from build123d import *

# Parameters (mm, degrees)
SKETCH1_W           = 60
SKETCH1_H           = 60
BOSS_EXTRUDE1_DEPTH = 5
SKETCH2_W           = 30
SKETCH2_H           = 14.2
SKETCH2_W_2         = 20.2
SKETCH2_H_2         = 8.2
BOSS_EXTRUDE2_DEPTH = 3
SKETCH3_W           = 20.2
SKETCH3_H           = 8.2
CUT_EXTRUDE1_DEPTH  = 15
SKETCH5_R           = 1
CUT_EXTRUDE2_DEPTH  = 15
FILLET1_R           = 2
SKETCH6_W           = 120.017280655
SKETCH6_H           = 101.423054075
CUT_EXTRUDE3_DEPTH  = 15
BOSS_EXTRUDE3_DEPTH = 5
CUT_EXTRUDE4_DEPTH  = 15
FILLET3_R           = 5
SKETCH9_R           = 1
CUT_EXTRUDE5_DEPTH  = 15
SKETCH10_R          = 1
CUT_EXTRUDE6_DEPTH  = 10
FILLET4_R           = 1


with BuildPart() as part:
    # Sketch1 → Boss-Extrude1 (new body)
    with BuildSketch(Plane.XY):
        with Locations((30, 30)):
            Rectangle(SKETCH1_W, SKETCH1_H)
    extrude(amount=BOSS_EXTRUDE1_DEPTH)

    # Sketch2 → Boss-Extrude2 (add)
    with BuildSketch(Plane.XY.offset(5)):
        with Locations((24, 30)):
            Rectangle(SKETCH2_W, SKETCH2_H)
        with Locations((24, 30)):
            Rectangle(SKETCH2_W_2, SKETCH2_H_2, mode=Mode.SUBTRACT)
    extrude(amount=BOSS_EXTRUDE2_DEPTH)

    # Sketch3 → Cut-Extrude1 (cut)
    with BuildSketch(Plane.XY.offset(5)):
        with Locations((24, 30)):
            Rectangle(SKETCH3_W, SKETCH3_H)
    extrude(amount=-CUT_EXTRUDE1_DEPTH, mode=Mode.SUBTRACT)

    # Sketch5 → Cut-Extrude2 (cut)
    with BuildSketch(Plane.XY.offset(8)):
        with Locations((12, 30)):
            Circle(SKETCH5_R)
        with Locations((36, 30)):
            Circle(SKETCH5_R)
    extrude(amount=-CUT_EXTRUDE2_DEPTH, mode=Mode.SUBTRACT)

    # Fillet1
    fillet1_edges = [part.edges().sort_by_distance(p)[0] for p in [
        (39, 22.9, 6.5),
        (39, 37.1, 6.5),
        (9, 37.1, 6.5),
        (9, 22.9, 6.5),
        (0, 0, 2.5),
        (0, 60, 2.5),
        (60, 60, 2.5),
        (60, 0, 2.5),
    ]]
    fillet(fillet1_edges, radius=FILLET1_R)

    # Sketch6 → Cut-Extrude3 (cut)
    with BuildSketch(Plane(origin=(0, 0, 0), x_dir=(-1, 0, 0), z_dir=(0, 0, -1))):
        with Locations((-31.690384235, 31.655167897)):
            Rectangle(SKETCH6_W, SKETCH6_H)
        Polygon((-8.786796564, 51.213203436), (12.426406871, 30), (-30, -12.426406871), (-72.426406871, 30), (-30, 72.426406871), align=None, mode=Mode.SUBTRACT)
    extrude(amount=-CUT_EXTRUDE3_DEPTH, mode=Mode.SUBTRACT)

    # Sketch7 → Boss-Extrude3 (add)
    with BuildSketch(Plane(origin=(0, 0, 0), x_dir=(-1, 0, 0), z_dir=(0, 0, -1))):
        Polygon((-8.786796564, 51.213203436), (12.426406871, 30), (-30, -12.426406871), (-72.426406871, 30), (-30, 72.426406871), align=None)
        Polygon((-19.393398282, 40.606601718), (-8.786796564, 30), (-30, 8.786796564), (-51.213203436, 30), (-30, 51.213203436), align=None, mode=Mode.SUBTRACT)
    extrude(amount=-BOSS_EXTRUDE3_DEPTH)

    # Sketch8 → Cut-Extrude4 (cut)
    with BuildSketch(Plane(origin=(0, 0, 0), x_dir=(-1, 0, 0), z_dir=(0, 0, -1))):
        Polygon((-30, -12.426406871), (12.426406871, 30), (-30, 72.426406871), (-72.426406871, 30), align=None)
        Polygon((-30, -5.355339059), (5.355339059, 30), (-30, 65.355339059), (-65.355339059, 30), align=None, mode=Mode.SUBTRACT)
    extrude(amount=-CUT_EXTRUDE4_DEPTH, mode=Mode.SUBTRACT)

    # Fillet3
    fillet3_edges = [part.edges().sort_by_distance(p)[0] for p in [
        (65.355339059, 30, 2.5),
        (30, 65.355339059, 2.5),
        (-5.355339059, 30, 2.5),
        (30, -5.355339059, 2.5),
    ]]
    fillet(fillet3_edges, radius=FILLET3_R)

    # Sketch9 → Cut-Extrude5 (cut)
    with BuildSketch(Plane(origin=(0, 0, 0), x_dir=(-1, 0, 0), z_dir=(0, 0, -1))):
        with Locations((-30, 58.284271247)):
            Circle(SKETCH9_R)
        with Locations((-30, 1.715728753)):
            Circle(SKETCH9_R)
        with Locations((-1.715728753, 30)):
            Circle(SKETCH9_R)
        with Locations((-58.284271247, 30)):
            Circle(SKETCH9_R)
    extrude(amount=-CUT_EXTRUDE5_DEPTH, mode=Mode.SUBTRACT)

    # Sketch10 → Cut-Extrude6 (cut)
    with BuildSketch(Plane(origin=(0, 0, 0), x_dir=(-1, 0, 0), z_dir=(0, 0, -1))):
        with Locations((-45.556349186, 45.556349186)):
            Circle(SKETCH10_R)
        with Locations((-45.556349186, 14.443650814)):
            Circle(SKETCH10_R)
        with Locations((-14.443650814, 14.443650814)):
            Circle(SKETCH10_R)
        with Locations((-14.443650814, 45.556349186)):
            Circle(SKETCH10_R)
    extrude(amount=-CUT_EXTRUDE6_DEPTH, mode=Mode.SUBTRACT)

    # Fillet4
    # the kernel refuses this fillet: 1 mm, written as the material it adds along each edge
    with BuildSketch(Plane(origin=(37, 35.1, 5), x_dir=(0, 1, 0), z_dir=(-1, 0, 0))) as fillet4_piece_1:
        with BuildLine():
            CenterArc((2 + FILLET4_R, -FILLET4_R), FILLET4_R, 90, 90)
            Line((2, -FILLET4_R), (2, 0))
            Line((2, 0), (2 + FILLET4_R, 0))
        make_face()
    revolve(axis=Axis((37, 35.1, 5), (0, 0, -1)), revolution_arc=90)
    with BuildSketch(Plane(origin=(37, 22.9, 5), x_dir=(0, -1, 0), z_dir=(-1, 0, 0)), Plane(origin=(11, 37.1, 5), x_dir=(0, 1, 0), z_dir=(1, 0, 0))) as fillet4_piece_2:
        with BuildLine():
            CenterArc((FILLET4_R, FILLET4_R), FILLET4_R, 180, 90)
            Line((0, FILLET4_R), (0, 0))
            Line((0, 0), (FILLET4_R, 0))
        make_face()
    extrude(amount=26)
    with BuildSketch(Plane(origin=(9, 24.9, 5), x_dir=(-1, 0, 0), z_dir=(0, 1, 0)), Plane(origin=(39, 35.1, 5), x_dir=(1, 0, 0), z_dir=(0, -1, 0))) as fillet4_piece_3:
        with BuildLine():
            CenterArc((FILLET4_R, FILLET4_R), FILLET4_R, 180, 90)
            Line((0, FILLET4_R), (0, 0))
            Line((0, 0), (FILLET4_R, 0))
        make_face()
    extrude(amount=10.2)
    with BuildSketch(Plane(origin=(11, 24.9, 5), x_dir=(0, -1, 0), z_dir=(1, 0, 0))) as fillet4_piece_4:
        with BuildLine():
            CenterArc((2 + FILLET4_R, -FILLET4_R), FILLET4_R, 90, 90)
            Line((2, -FILLET4_R), (2, 0))
            Line((2, 0), (2 + FILLET4_R, 0))
        make_face()
    revolve(axis=Axis((11, 24.9, 5), (0, 0, -1)), revolution_arc=90)
    with BuildSketch(Plane(origin=(11, 35.1, 5), x_dir=(0, 1, 0), z_dir=(1, 0, 0))) as fillet4_piece_5:
        with BuildLine():
            CenterArc((2 + FILLET4_R, FILLET4_R), FILLET4_R, 180, 90)
            Line((2, FILLET4_R), (2, 0))
            Line((2, 0), (2 + FILLET4_R, 0))
        make_face()
    revolve(axis=Axis((11, 35.1, 5), (0, 0, 1)), revolution_arc=90)
    with BuildSketch(Plane(origin=(37, 24.9, 5), x_dir=(1, 0, 0), z_dir=(0, 1, 0))) as fillet4_piece_6:
        with BuildLine():
            CenterArc((2 + FILLET4_R, -FILLET4_R), FILLET4_R, 90, 90)
            Line((2, -FILLET4_R), (2, 0))
            Line((2, 0), (2 + FILLET4_R, 0))
        make_face()
    revolve(axis=Axis((37, 24.9, 5), (0, 0, -1)), revolution_arc=90)
    # the kernel refuses this fillet: 1 mm, written as the material it takes off along each edge
    with BuildSketch(Plane(origin=(34.1, 25.9, 8), x_dir=(0, 0, -1), z_dir=(0, 1, 0)), Plane(origin=(13.9, 34.1, 8), x_dir=(0, 0, -1), z_dir=(0, -1, 0))) as fillet4_2_piece_1:
        with BuildLine():
            CenterArc((FILLET4_R, -FILLET4_R), FILLET4_R, 90, 90)
            Line((0, -FILLET4_R), (0, 0))
            Line((0, 0), (FILLET4_R, 0))
        make_face()
    extrude(amount=8.2, mode=Mode.SUBTRACT)
    with BuildSketch(Plane(origin=(34.1, 34.1, 8), x_dir=(0, 0, -1), z_dir=(-1, 0, 0)), Plane(origin=(13.9, 25.9, 8), x_dir=(0, 0, -1), z_dir=(1, 0, 0))) as fillet4_2_piece_2:
        with BuildLine():
            CenterArc((FILLET4_R, -FILLET4_R), FILLET4_R, 90, 90)
            Line((0, -FILLET4_R), (0, 0))
            Line((0, 0), (FILLET4_R, 0))
        make_face()
    extrude(amount=20.2, mode=Mode.SUBTRACT)
    with BuildSketch(Plane(origin=(13.9, 25.9, 8), x_dir=(0, 0, -1), z_dir=(1, 0, 0))) as fillet4_2_piece_3a_section:
        with BuildLine():
            CenterArc((FILLET4_R, -FILLET4_R), FILLET4_R, 90, 90)
            Line((0, -FILLET4_R), (0, 0))
            Line((0, 0), (FILLET4_R, 0))
        make_face()
    fillet4_2_piece_3a = extrude(amount=22.7, mode=Mode.PRIVATE)
    fillet4_2_piece_3a = split(fillet4_2_piece_3a, bisect_by=Plane(origin=(34.1, 25.673604886, 7.773604886), z_dir=(1, 0, 0)), keep=Keep.TOP, mode=Mode.PRIVATE)
    with BuildSketch(Plane(origin=(34.1, 23.4, 8), x_dir=(0, 0, -1), z_dir=(0, 1, 0))) as fillet4_2_piece_3b_section:
        with BuildLine():
            CenterArc((FILLET4_R, -FILLET4_R), FILLET4_R, 90, 90)
            Line((0, -FILLET4_R), (0, 0))
            Line((0, 0), (FILLET4_R, 0))
        make_face()
    fillet4_2_piece_3b = extrude(amount=10.7, mode=Mode.PRIVATE)
    fillet4_2_piece_3b = split(fillet4_2_piece_3b, bisect_by=Plane(origin=(34.326395114, 25.9, 7.773604886), z_dir=(0, -1, 0)), keep=Keep.TOP, mode=Mode.PRIVATE)
    fillet4_2_piece_3 = fillet4_2_piece_3a & fillet4_2_piece_3b
    add(fillet4_2_piece_3, mode=Mode.SUBTRACT)
    with BuildSketch(Plane(origin=(34.1, 25.9, 8), x_dir=(0, 0, -1), z_dir=(0, 1, 0))) as fillet4_2_piece_4a_section:
        with BuildLine():
            CenterArc((FILLET4_R, -FILLET4_R), FILLET4_R, 90, 90)
            Line((0, -FILLET4_R), (0, 0))
            Line((0, 0), (FILLET4_R, 0))
        make_face()
    fillet4_2_piece_4a = extrude(amount=10.7, mode=Mode.PRIVATE)
    fillet4_2_piece_4a = split(fillet4_2_piece_4a, bisect_by=Plane(origin=(34.326395114, 34.1, 7.773604886), z_dir=(0, 1, 0)), keep=Keep.TOP, mode=Mode.PRIVATE)
    with BuildSketch(Plane(origin=(36.6, 34.1, 8), x_dir=(0, 0, -1), z_dir=(-1, 0, 0))) as fillet4_2_piece_4b_section:
        with BuildLine():
            CenterArc((FILLET4_R, -FILLET4_R), FILLET4_R, 90, 90)
            Line((0, -FILLET4_R), (0, 0))
            Line((0, 0), (FILLET4_R, 0))
        make_face()
    fillet4_2_piece_4b = extrude(amount=22.7, mode=Mode.PRIVATE)
    fillet4_2_piece_4b = split(fillet4_2_piece_4b, bisect_by=Plane(origin=(34.1, 34.326395114, 7.773604886), z_dir=(1, 0, 0)), keep=Keep.TOP, mode=Mode.PRIVATE)
    fillet4_2_piece_4 = fillet4_2_piece_4a & fillet4_2_piece_4b
    add(fillet4_2_piece_4, mode=Mode.SUBTRACT)
    with BuildSketch(Plane(origin=(13.9, 36.6, 8), x_dir=(0, 0, -1), z_dir=(0, -1, 0))) as fillet4_2_piece_5a_section:
        with BuildLine():
            CenterArc((FILLET4_R, -FILLET4_R), FILLET4_R, 90, 90)
            Line((0, -FILLET4_R), (0, 0))
            Line((0, 0), (FILLET4_R, 0))
        make_face()
    fillet4_2_piece_5a = extrude(amount=10.7, mode=Mode.PRIVATE)
    fillet4_2_piece_5a = split(fillet4_2_piece_5a, bisect_by=Plane(origin=(13.673604886, 34.1, 7.773604886), z_dir=(0, 1, 0)), keep=Keep.TOP, mode=Mode.PRIVATE)
    with BuildSketch(Plane(origin=(34.1, 34.1, 8), x_dir=(0, 0, -1), z_dir=(-1, 0, 0))) as fillet4_2_piece_5b_section:
        with BuildLine():
            CenterArc((FILLET4_R, -FILLET4_R), FILLET4_R, 90, 90)
            Line((0, -FILLET4_R), (0, 0))
            Line((0, 0), (FILLET4_R, 0))
        make_face()
    fillet4_2_piece_5b = extrude(amount=22.7, mode=Mode.PRIVATE)
    fillet4_2_piece_5b = split(fillet4_2_piece_5b, bisect_by=Plane(origin=(13.9, 34.326395114, 7.773604886), z_dir=(-1, 0, 0)), keep=Keep.TOP, mode=Mode.PRIVATE)
    fillet4_2_piece_5 = fillet4_2_piece_5a & fillet4_2_piece_5b
    add(fillet4_2_piece_5, mode=Mode.SUBTRACT)
    with BuildSketch(Plane(origin=(11.4, 25.9, 8), x_dir=(0, 0, -1), z_dir=(1, 0, 0))) as fillet4_2_piece_6a_section:
        with BuildLine():
            CenterArc((FILLET4_R, -FILLET4_R), FILLET4_R, 90, 90)
            Line((0, -FILLET4_R), (0, 0))
            Line((0, 0), (FILLET4_R, 0))
        make_face()
    fillet4_2_piece_6a = extrude(amount=22.7, mode=Mode.PRIVATE)
    fillet4_2_piece_6a = split(fillet4_2_piece_6a, bisect_by=Plane(origin=(13.9, 25.673604886, 7.773604886), z_dir=(-1, 0, 0)), keep=Keep.TOP, mode=Mode.PRIVATE)
    with BuildSketch(Plane(origin=(13.9, 34.1, 8), x_dir=(0, 0, -1), z_dir=(0, -1, 0))) as fillet4_2_piece_6b_section:
        with BuildLine():
            CenterArc((FILLET4_R, -FILLET4_R), FILLET4_R, 90, 90)
            Line((0, -FILLET4_R), (0, 0))
            Line((0, 0), (FILLET4_R, 0))
        make_face()
    fillet4_2_piece_6b = extrude(amount=10.7, mode=Mode.PRIVATE)
    fillet4_2_piece_6b = split(fillet4_2_piece_6b, bisect_by=Plane(origin=(13.673604886, 25.9, 7.773604886), z_dir=(0, -1, 0)), keep=Keep.TOP, mode=Mode.PRIVATE)
    fillet4_2_piece_6 = fillet4_2_piece_6a & fillet4_2_piece_6b
    add(fillet4_2_piece_6, mode=Mode.SUBTRACT)


solid = part.part
Input: part model. Units: mm. Frame: model coordinates. A direction names the side the tool comes from. Coordinates: 2 decimals unless noted, no trailing zeros. Loops run counter-clockwise (first coordinate to the right, second up) from the corner with the lowest first, then second, coordinate; pieces in that order, holes last.
(1) Section D-D on y = 12. Return the cut outline in (x, z), then the cut area to 3 significant figures.
(2) Set-up query: faces 5 (the face through (24, 22.9, 7)), 6 (the face through (9.6, 36.53, 7.01)), 7 (the face through (24, 34.1, 3)), 8 (the face through (38.4, 23.47, 7.01)). Return all of +Z, -Z, +X, -X, +Y, -Y with unobstructed straight access to the full face (end or side cutting, diameter ignored); none if empty.
(3) Material intervals for probe 1 along X at (y, z) = (30, 6.25); probe 2 along Y at (x, z) = (15, 6.5); probe 3 along Z at (x, y) = (17, 43), sorted ascending.
(4) Section A-A on x = 30. Return the cut outline in (y, z).
(5) Section B-B on z = 3.25. Count the separate pieces of the cut face and the enclosed holes in it, then the cut area to 3 significant figures.
(6) First-contact query: pin 1 Ø1.5 at (x, z) = (28, 5) entering from +Y; pin 2 Ø3.5 at (y, z) = (30.5, 3.5) entering from -X; pin 3 Ø1 at (x, y) = (53.5, 32.5) entering from +Z; pin 4 Ø1.6 at (x, z) = (18, 7) entering from -Y. Flat tips, straight axial feed; report the tip coordinate or a pass-through.
(7) Pull-direction query (X, two-part tool) for faces 1 (the face through (63.284, 30.055, 2.535)), 2 (the face through (12.52, 12.124, 2.465)), 3 (the face through (24, 24, 8)), 4 (the face through (46.555, 45.6, 2.465)); classes: released by +X, released by -X, zero draft, split by the parting line, or undercut.
(8) Section C-C on x = 12. Return the cut outline in (y, z).
Data:
1. outline: (12.64, 0) - (47.36, 0) - (47.36, 5) - (12.64, 5) - close
1. area: 174 mm2
2. face 5: +Z, +X, -X, -Y
2. face 6: +Z, -X, +Y
2. face 7: +Z, -Z
2. face 8: +Z, +X, -Y
3. probe 1: x = 9 to 11, 13 to 13.9, 34.1 to 35, 37 to 39
3. probe 2: y = 22.9 to 25.9, 34.1 to 37.1
3. probe 3: z = 0 to 5
4. outline: (-3.28, 0) - (0.72, 0) - (0.72, 5) - (-3.28, 5) - close; (2.72, 0) - (25.9, 0) - (25.9, 7) arc R1 ccw to (24.9, 8) - (22.9, 8) - (22.9, 6) arc R1 cw to (21.9, 5) - (2.72, 5) - close; (34.1, 0) - (57.28, 0) - (57.28, 5) - (38.1, 5) arc R1 cw to (37.1, 6) - (37.1, 8) - (35.1, 8) arc R1 ccw to (34.1, 7) - close; (59.28, 0) - (63.28, 0) - (63.28, 5) - (59.28, 5) - close
5. separate pieces: 1
5. enclosed holes: 11
5. area: 2,280 mm2
6. pin 1: stops at y = 63.13
6. pin 2: stops at x = -3.28
6. pin 3: stops at z = 5
6. pin 4: stops at y = 22.9
7. face 1: released by +X
7. face 2: released by -X
7. face 3: zero draft
7. face 4: undercut
8. outline: (12.64, 0) - (29, 0) - (29, 8) - (22.9, 8) - (22.9, 6) arc R1 cw to (21.9, 5) - (12.64, 5) - close; (31, 0) - (47.36, 0) - (47.36, 5) - (38.1, 5) arc R1 cw to (37.1, 6) - (37.1, 8) - (31, 8) - close
